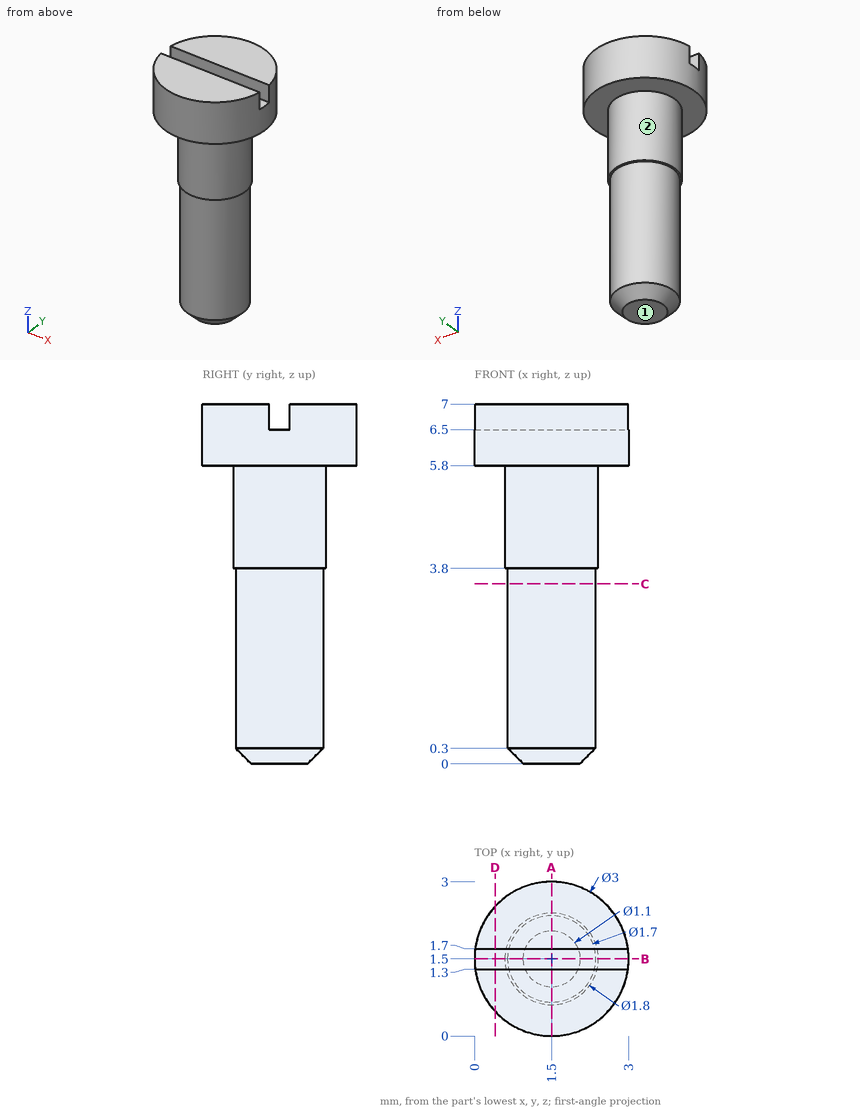
Can you work these out from the drawing? Everything is in mm from the part's minimum corner. A direction names the side the tool comes from. Give positions to 0.01 mm unless a question says otherwise; leave off trailing zeros. Loops run counter-clockwise (first coordinate to the right, second up) from the corner with the lowest first, then second, coordinate; pieces in that order, holes last. Notation, with made-up numbers: M -21,-16 L 4,-16 A20 ccw 4,3 Z; hole C 40,2 d6. An arc over 180 degrees is marked long. Use CSV: the item, a comma, the result in double quotes. Start each with the question number.
1. Imagine slicing it at A-A, the plane x = 1.5. Write out the boundary of the cut face in (y, z).
2. Imagine slicing it at B-B, the plane y = 1.5. Write out the boundary of the cut face in (x, z).
3. Imagine slicing it at D-D, the plane x = 0.4. Write out the boundary of the cut face in (y, z), plus the area to 3 significant figures.
4. If I drill on L1, parallel to Z at x = 2.5, y = 2.35; L2, parallel to Z at x = 2.65, y = 1.55; L3, parallel to Y at x = 1.55, z = 5.75, over which ranges is the centre line in solid material (lowest first)?
5. For P1, Ø1, axis at x = 1, y = 1, coming from the -Z side; P2, Ø1.5, axis at x = 1, z = 4, coming from the -Y side; P3, Ø1, axis at x = 0.5, z = 2, coming from the -Y side, each with a flat end and sliding along its axis, tell me the tip position at first contact or that it passes through.
6. Imagine slicing it at C-C, the plane z = 3.5. Write out the boundary of the cut face in (x, y), plus the area to 3 significant figures.
7. On a 3-axis mill with a long thin cutter (end or side, diameter ignored), from which of +Z, -Z, +X, -X, +Y, -Y can I reach the whole of each face in a straight line? I mean the marked faces 1 and 2. Say none if no direction works.
Response values:
1,outline,"M 0,5.8 L 0.6,5.8 L 0.6,3.8 L 0.65,3.8 L 0.65,0.3 L 0.95,0 L 2.05,0 L 2.35,0.3 L 2.35,3.8 L 2.4,3.8 L 2.4,5.8 L 3,5.8 L 3,7 L 1.7,7 L 1.7,6.5 L 1.3,6.5 L 1.3,7 L 0,7 Z"
2,outline,"M 0,5.8 L 0.6,5.8 L 0.6,3.8 L 0.65,3.8 L 0.65,0.3 L 0.95,0 L 2.05,0 L 2.35,0.3 L 2.35,3.8 L 2.4,3.8 L 2.4,5.8 L 3,5.8 L 3,6.5 L 0,6.5 Z"
3,outline,"M 0.48,5.8 L 2.52,5.8 L 2.52,7 L 1.7,7 L 1.7,6.5 L 1.3,6.5 L 1.3,7 L 0.48,7 Z"
3,area,"2.25 mm^2"
4,L1,"5.8 to 7"
4,L2,"5.8 to 6.5"
4,L3,"0.6 to 2.4"
5,P1,"z = 0"
5,P2,"y = 0.6"
5,P3,"y = 0.81"
6,outline,"C 1.5,1.5 d1.7"
6,area,"2.27 mm^2"
7,face 1,"-Z, +X, -X, +Y, -Y"
7,face 2,"-Z"
